from build123d import *

# Parameters (mm, degrees)
F1_DEPTH = 50.8
F3_DEPTH = 86.868
F5_DEPTH = 97.028
F6_SIZE  = 5.08


with BuildPart() as f1:
    # F0 (on Front) → F1 (new body)
    with BuildSketch(Plane.XZ):
        Polygon((-14.398527, 25.359184), (-76.246753, 0), (-17.016442, -27.980816), (42.541102, -27.980816), (42.541102, 25.359184), align=None)
    extrude(amount=F1_DEPTH)

    # F2 (on Right) → F3 (join)
    with BuildSketch(Plane.YZ):
        Polygon((-11.453375, 25.031945), (-38.614232, 25.031945), (-50.722085, 6.706545), (-50.722085, -12.600573), (-38.614232, -27.653579), (-11.453375, -27.653579), (0, -12.600573), (0, 6.706545), align=None)
    extrude(amount=F3_DEPTH)

    # F4 (on face) → F5 (cut)
    with BuildSketch(Plane.XY.offset(25.359184)):
        with BuildLine():
            Line((28.871851, -16.200203), (0, -16.200203))
            ThreePointArc((0, -16.200203), (-7.853743, -24.053946), (0, -31.907689))
            Line((0, -31.907689), (28.871851, -31.907689))
            ThreePointArc((28.871851, -31.907689), (36.725594, -24.053946), (28.871851, -16.200203))
        make_face()
    extrude(amount=-F5_DEPTH, mode=Mode.SUBTRACT)

    # F6
    f6_edges = [f1.edges().sort_by_distance(p)[0] for p in [
        (86.868, -25.033804, 25.031945),
        (86.868, -5.726688, 15.869245),
        (86.868, 0, -2.947014),
        (86.868, -5.726688, -20.127076),
        (86.868, -25.033804, -27.653579),
        (86.868, -44.668159, 15.869245),
        (86.868, -50.722085, -2.947014),
        (86.868, -44.668159, -20.127076),
    ]]
    chamfer(f6_edges, length=F6_SIZE)


solid = f1.part
The listing builds one solid part. Answer for the finished solid, in the listing's coordinates (mm). A direction names the side the tool comes from. Give positions to 0.01 mm unless a question says otherwise; leave off trailing zeros. Write each loop counter-clockwise with the first axis right and the second up, starting at its lowest first coordinate (ties: lowest second). Pieces come first, ordered by that corner, then holes. Notation, with made-up numbers: (21.5, -2) -> (36.5, -2) arc R6 cw to (36.5, 7) -> close; hole circle Ø4 at (44, 84.5). An arc over 180 degrees is marked (long way). One line per question, with ' | ' between items. Start each with the question number.
1. Find the intervals of material crossed by probe 1 along Y at (x, z) = (-0.5, 7); probe 2 along Y at (x, z) = (48, 2); probe 3 along Z at (x, y) = (53, -18.5), in increasing order.
2. For faces 4 (the flat face through (61.89, -5.807, -20.232)), 5 (the flat face through (14, -31.908, -1)), 6 (the flat face through (61.89, -44.58, 16)), 7 (the flat face through (62, -25, -27.654)), determine the directions among +Z, -Z, +X, -X, +Y, -Y from which every point of the face is accessible in a straight line to the end or side of a thin tool.
3. Section D-D (y = -30) is taken. Determine the outline of the cut face in (x, z).
4. Given pin 1 Ø15.5 at (x, z) = (57, -5) entering from -Y; pin 2 Ø13.5 at (x, y) = (67.5, -27.5) entering from -Z; pin 3 Ø2 at (y, z) = (-45.5, 10.5) entering from -X, each flat-ended and moving along its own axis, determine where each tip first touches the part or whether it passes through.
5. For a pull along Y with two mould halves and no side action, classify faces 1 (the cylindrical face through (36.724, -24.227, -0.937)), 2 (the flat face through (14, -36, 25.359)), 3 (the flat face through (-4, -50.8, -1)) as pulls with the +Y half, pulls with the -Y half, needs draft (parallel to the pull), parting line crosses it, or undercut.
6. Section A-A (x = 21) is taken. Determine the outline of the cut face in (y, z), plus the area to 3 significant figures.
7. Section C-C (x = 69) is taken. Determine the outline of the cut face in (y, z).
8. Section B-B (z = 13.5) is taken. Determine the outline of the cut face in (x, y).
Response values:
1) probe 1: -50.8 to -31.89, -16.22 to 0 | probe 2: -50.72 to 0 | probe 3: -27.65 to 25.03
2) face 4: -Z, +X, +Y | face 5: +Z, -Z | face 6: +Z, +X, -Y | face 7: -Z, +X, +Y, -Y
3) outline: (-76.25, 0) -> (-17.02, -27.98) -> (-5.13, -27.98) -> (-5.13, 25.36) -> (-14.4, 25.36) -> close; (34, -27.98) -> (42.54, -27.98) -> (42.54, -27.65) -> (81.79, -27.65) -> (86.87, -22.57) -> (86.87, 19.95) -> (81.79, 25.03) -> (42.54, 25.03) -> (42.54, 25.36) -> (34, 25.36) -> close
4) pin 1: y = -50.72 | pin 2: z = -27.65 | pin 3: x = -53.08
5) face 1: undercut | face 2: needs draft | face 3: pulls with the -Y half
6) outline: (-50.8, -27.98) -> (-31.91, -27.98) -> (-31.91, 25.36) -> (-50.8, 25.36) -> close; (-16.2, -27.98) -> (0, -27.98) -> (0, 25.36) -> (-16.2, 25.36) -> close | area: 1,870 mm2
7) outline: (-50.72, -12.6) -> (-38.61, -27.65) -> (-11.45, -27.65) -> (0, -12.6) -> (0, 6.71) -> (-11.45, 25.03) -> (-38.61, 25.03) -> (-50.72, 6.71) -> close
8) outline: (-43.32, -50.8) -> (42.54, -50.8) -> (42.54, -46.23) -> (81.79, -46.23) -> (86.87, -40.14) -> (86.87, -10.24) -> (81.79, -4.25) -> (42.54, -4.25) -> (42.54, 0) -> (-43.32, 0) -> close; hole (0, -31.91) -> (28.87, -31.91) arc R7.85 ccw to (28.87, -16.2) -> (0, -16.2) arc R7.85 ccw to start
